from build123d import *

# Parameters (mm, degrees)
F0_W      = 9
F0_H      = 89
F2_R      = 9
F3_DEPTH  = 5
F4_R      = 3
F5_R      = 7
F6_DEPTH  = 11
F8_DEPTH  = 11
F10_R     = 3.9621233683
F11_DEPTH = 18
F9_R      = 9.1436864808
F12_DEPTH = 15


with BuildPart() as f1:
    # F0 (on Front) → F1 (revolve)
    with BuildSketch(Plane.XZ):
        with Locations((4.5, 44.5)):
            Rectangle(F0_W, F0_H)
    revolve(axis=Axis((0, 0, 44.5), (0, 0, -1)))

    # F2 (on face) → F3 (join)
    with BuildSketch(Plane.XY.offset(89)):
        Circle(F2_R)
    extrude(amount=F3_DEPTH)

    # F4
    f4_edges = [f1.edges().sort_by_distance(p)[0] for p in [
        (-9, 0, 94),
    ]]
    fillet(f4_edges, radius=F4_R)

    # F5 (on face) → F6 (cut)
    with BuildSketch(Plane(origin=(0, 0, 0), x_dir=(1, 0, 0), z_dir=(0, 0, -1))):
        Circle(F5_R)
    extrude(amount=-F6_DEPTH, mode=Mode.SUBTRACT)

    # F7 (on face) → F8 (join)
    with BuildSketch(Plane(origin=(0, 0, 11), x_dir=(1, 0, 0), z_dir=(0, 0, -1))):
        with BuildLine():
            Line((-0.5, 5), (0, 5))
            Line((0, 5), (0.5, 5))
            Line((0.5, 5), (0.5, 6.9821200219))
            ThreePointArc((0.5, 6.9821200219), (0, 7), (-0.5, 6.9821200219))
            Line((-0.5, 6.9821200219), (-0.5, 5))
        make_face()
        with BuildLine():
            ThreePointArc((7, 0), (6.9955285774, 0.2501597957), (6.9821200219, 0.5))
            Line((6.9821200219, 0.5), (5, 0.5))
            Line((5, 0.5), (5, 0))
            Line((5, 0), (5, -0.5))
            Line((5, -0.5), (6.9821200219, -0.5))
            ThreePointArc((6.9821200219, -0.5), (6.9955285774, -0.2501597957), (7, 0))
        make_face()
        with BuildLine():
            Line((-5, 0.5), (-6.9821200219, 0.5))
            ThreePointArc((-6.9821200219, 0.5), (-7, 0), (-6.9821200219, -0.5))
            Line((-6.9821200219, -0.5), (-5, -0.5))
            Line((-5, -0.5), (-5, 0))
            Line((-5, 0), (-5, 0.5))
        make_face()
        with BuildLine():
            Line((-0.5, -5), (-0.5, -6.9821200219))
            ThreePointArc((-0.5, -6.9821200219), (0, -7), (0.5, -6.9821200219))
            Line((0.5, -6.9821200219), (0.5, -5))
            Line((0.5, -5), (0, -5))
            Line((0, -5), (-0.5, -5))
        make_face()
    extrude(amount=F8_DEPTH)

    # F10 (on face) → F11 (join)
    with BuildSketch(Plane.XY.offset(94)):
        Circle(F10_R)
    extrude(amount=F11_DEPTH)

    # F9 (on face) → F12 (join)
    with BuildSketch(Plane.XY.offset(94)):
        Circle(F9_R)
    extrude(amount=F12_DEPTH)


solid = f1.part
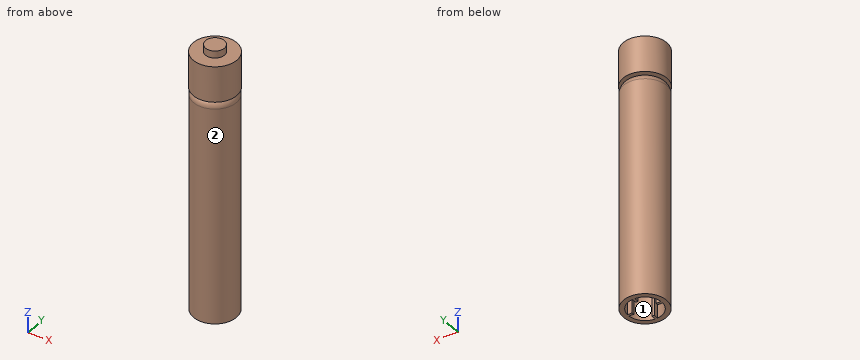
Read the model definition and answer for the solid it produces. Units are mm, in the model's axes. Face numbers are marked on the shaded views. Coordinates: 2 decimals unless noted, no trailing zeros. Order: outer loops, then holes, each group sorted by start corner. A loop starts at its lowest first (then second) coordinate and runs counter-clockwise, first axis right, second up. Notation, with made-up numbers: (-38, -23.75) -> (-7, -23.75) arc R30 ccw to (-7, 5.25) -> close; hole circle Ø6 at (-32.5, -39.5). An arc over 180 degrees is marked (long way). Answer as a JSON object with one key per item and string values.
1) A cutting plane is placed at C-C, the plane z = 37. Determine the outline of the cut face in (x, y), plus the area to 3 significant figures.
Model answer:
{"outline": "circle Ø18 at (0, 0)", "area": "254 mm²"}
2) Each of these flat-tipped pins is pushed along its axis until it touches: pin 1 (0.5 mm diameter, centred on y = 0, z = 4.5, fed in from -X); pin 2 (5 mm diameter, centred on x = -4, y = -6, fed in from +Z); pin 3 (1.6 mm diameter, centred on y = 5.5, z = 3, fed in from +X); pin 4 (3 mm diameter, centred on x = -7, y = -4.5, fed in from -Z). Where does it stop, or does it pass through?
Model answer:
{"pin 1": "stops at x = -9", "pin 2": "stops at z = 109", "pin 3": "stops at x = 7.68", "pin 4": "stops at z = 0"}
3) A cutting plane is placed at A-A, the plane z = 8. Determine the outline of the cut face in (x, y).
Model answer:
{"outline": "circle Ø18 at (0, 0); hole (-6.98, -0.5) arc R7 ccw to (-0.5, -6.98) -> (-0.5, -5) -> (0.5, -5) -> (0.5, -6.98) arc R7 ccw to (6.98, -0.5) -> (5, -0.5) -> (5, 0.5) -> (6.98, 0.5) arc R7 ccw to (0.5, 6.98) -> (0.5, 5) -> (-0.5, 5) -> (-0.5, 6.98) arc R7 ccw to (-6.98, 0.5) -> (-5, 0.5) -> (-5, -0.5) -> close"}
4) A cutting plane is placed at B-B, the plane z = 96.5. Determine the outline of the cut face in (x, y), plus the area to 3 significant figures.
Model answer:
{"outline": "circle Ø18.29 at (0, 0)", "area": "263 mm²"}
5) Consider line 1 along X through (y, z) = (0.5, 86); line 2 along Y through (x, z) = (6, 5); line 3 along Y through (x, z) = (-0.25, 65.5). Determine where each line is inside the solid, lowest interval first. Write a range as from..to.
Model answer:
{"line 1": "x = -8.99..8.99", "line 2": "y = -6.71..-3.61, -0.5..0.5, 3.61..6.71", "line 3": "y = -9..9"}
6) The mould has two halves that part along Y. Classify the marked faces 1 and 2: released by +Y, released by -Y, zero draft, split by the parting line, or undercut.
Model answer:
{"face 1": "undercut", "face 2": "split by the parting line"}
